Source: CAD feature listing. Evaluate the final solid. Frame: model axes, mm. A direction names the side the tool comes from. Give positions to 0.01 mm unless a question says otherwise; leave off trailing zeros. Order: outer loops, then holes, each group sorted by start corner. A loop starts at its lowest first (then second) coordinate and runs counter-clockwise, first axis right, second up. Notation, with made-up numbers: (-3.75, -8.75) - (7.25, -8.75) arc R16 ccw to (7.25, 21.25) - close; hole circle Ø5 at (78.5, 48). An arc over 180 degrees is marked (long way). One line per item, written item: value. Start each with the question number.
from build123d import *

# Parameters (mm, degrees)
F0_R     = 50.8
F1_DEPTH = 254
F2_T     = -2.54
F3_R     = 22.9273232768
F4_DEPTH = 152.908
F5_R     = 22.9235
F6_DEPTH = 92.202


with BuildPart() as f1:
    # F0 (on Top) → F1 (new body)
    with BuildSketch(Plane.XY):
        Circle(F0_R)
    extrude(amount=F1_DEPTH)

    # F2 (hollow: no face is removed)
    offset(amount=F2_T, mode=Mode.SUBTRACT)

    # F3 (on Front) → F4 (cut)
    with BuildSketch(Plane.XZ):
        with Locations((0, 190.627977252)):
            Circle(F3_R)
    extrude(amount=F4_DEPTH, mode=Mode.SUBTRACT)

    # F5 (on Front) → F6 (cut)
    with BuildSketch(Plane.XZ):
        with Locations((0, 77.4756367312)):
            Circle(F5_R)
    extrude(amount=F6_DEPTH, mode=Mode.SUBTRACT)


solid = f1.part
1. Section A-A on x = 0. Return the cut outline in (y, z), then the cut area to 3 significant figures.
2. Contact query for flat-ended pins moving along their axis: pin 1 Ø1 at (x, y) = (-8, -39) entering from -Z; pin 2 Ø2 at (x, z) = (-16, 207.5) entering from +Y; pin 3 Ø2 at (y, z) = (-24, 160) entering from +X; pin 4 Ø5 at (y, z) = (-7.5, 140.5) entering from +X. Output: stop coordinate, or through.
3. Section B-B on y = 0. Return the cut outline in (x, z).
4. Section D-D on z = 44.5. Return the cut outline in (x, y), then the cut area to 3 significant figures.
5. Set-up query: faces 1 (the cylindrical face through (25.944, 40.693, 125.258)), 2 (the cylindrical face through (15.97, -46.31, 93.92)), 3 (the flat face through (-1, 1, 0)). Return all of +Z, -Z, +X, -X, +Y, -Y with unobstructed straight access to the full face (end or side cutting, diameter ignored); none if empty.
6. Ray query, L1, parallel to Z at x = 16, y = -3; L2, parallel to Y at x = 0, z = 113; L3, parallel to X at y = -21, z = 20. Return the intervals inside material, ascending.
7. Section C-C on x = -31. Return the cut outline in (y, z).
8. Draft query along X for faces 4 (the flat face through (-1, 1, 254)), 5 (the cylindrical face through (15.98, -46.3, 207.07)), 6 (the cylindrical face through (-6.61, 50.37, 125.22)). Return one class per face: pulls with the +X half, pulls with the -X half, needs draft (parallel to the pull), parting line crosses it, or undercut.
Data:
1. outline: (-50.8, 0) - (50.8, 0) - (50.8, 254) - (-50.8, 254) - (-50.8, 213.56) - (-48.26, 213.56) - (-48.26, 251.46) - (48.26, 251.46) - (48.26, 2.54) - (-48.26, 2.54) - (-48.26, 54.55) - (-50.8, 54.55) - close; (-50.8, 100.4) - (-48.26, 100.4) - (-48.26, 167.7) - (-50.8, 167.7) - close
1. area: 1,550 mm2
2. pin 1: stops at z = 0
2. pin 2: stops at y = 48.53
2. pin 3: stops at x = 45.3
2. pin 4: stops at x = 50.55
3. outline: (-50.8, 0) - (50.8, 0) - (50.8, 254) - (-50.8, 254) - close; hole (-48.26, 2.54) - (48.26, 2.54) - (48.26, 251.46) - (-48.26, 251.46) - close
4. outline: circle Ø101.6 at (0, 0); hole circle Ø96.52 at (0, 0)
4. area: 790 mm2
5. face 1: none
5. face 2: -Y
5. face 3: -Z, +X, -X, +Y, -Y
6. L1: z = 0 to 2.54, 251.46 to 254
6. L2: y = -50.8 to -48.26, 48.26 to 50.8
6. L3: x = -46.26 to -43.45, 43.45 to 46.26
7. outline: (-40.24, 0) - (40.24, 0) - (40.24, 254) - (-40.24, 254) - close; hole (-36.99, 2.54) - (36.99, 2.54) - (36.99, 251.46) - (-36.99, 251.46) - close
8. face 4: needs draft
8. face 5: undercut
8. face 6: parting line crosses it
